Read the model definition and answer for the solid it produces. Units are mm, in the model's axes. A direction names the side the tool comes from. Give positions to 0.01 mm unless a question says otherwise; leave off trailing zeros. Order: outer loops, then holes, each group sorted by start corner. A loop starts at its lowest first (then second) coordinate and runs counter-clockwise, first axis right, second up.
```python
from build123d import *

# Parameters (mm, degrees)
F0_R      = 5.6261
F1_DEPTH  = 12.7
F2_R      = 5.6007
F3_DEPTH  = 9.525
F4_R      = 12.7
F4_R_2    = 5.6007
F6_DEPTH  = 6.35
F7_DEPTH  = 6.35
F8_R      = 7.62
F9_DEPTH  = 6.35
F10_DEPTH = 6.35
F11_R     = 1.27


with BuildPart() as f1:
    # F0 (on Top) → F1 (new body)
    with BuildSketch(Plane.XY):
        Circle(F0_R)
    extrude(amount=F1_DEPTH)

    # F2 (on face) → F3 (join)
    with BuildSketch(Plane.XY.offset(12.7)):
        Circle(F2_R)
    extrude(amount=F3_DEPTH)

    # F4 (on face) → F6 (join)
    with BuildSketch(Plane.XY.offset(22.225)):
        Circle(F4_R)
        Circle(F4_R_2, mode=Mode.SUBTRACT)
    extrude(amount=F6_DEPTH)

    # F7 (add): a face of the model
    f7_faces = [f1.faces().sort_by_distance(p)[0] for p in [
        (0, 0, 22.225),
    ]]
    extrude(f7_faces, amount=F7_DEPTH)

    # F8 (on face) → F9 (join)
    with BuildSketch(Plane(origin=(0, 0, 22.225), x_dir=(1, 0, 0), z_dir=(0, 0, -1))):
        Circle(F8_R)
    extrude(amount=F9_DEPTH)

    # F5 (on face) → F10 (join)
    with BuildSketch(Plane.XY.offset(22.225)):
        with BuildLine():
            ThreePointArc((-6.35, -10.9985226281), (-10.9985226281, -6.35), (-12.7, 0))
            Line((-12.7, 0), (-29.197504538, -9.524838686))
            ThreePointArc((-29.197504538, -9.524838686), (-27.4960271661, -15.874838686), (-22.847504538, -20.523361314))
            Line((-22.847504538, -20.523361314), (-6.35, -10.9985226281))
        make_face()
        with BuildLine():
            Line((-6.35, 30.0482), (-6.35, 10.9985226281))
            ThreePointArc((-6.35, 10.9985226281), (0, 12.7), (6.35, 10.9985226281))
            Line((6.35, 10.9985226281), (6.35, 30.0482))
            ThreePointArc((6.35, 30.0482), (0, 31.7496773719), (-6.35, 30.0482))
        make_face()
        with BuildLine():
            Line((29.197504538, -9.524838686), (12.7, 0))
            ThreePointArc((12.7, 0), (10.9985226281, -6.35), (6.35, -10.9985226281))
            Line((6.35, -10.9985226281), (22.847504538, -20.523361314))
            ThreePointArc((22.847504538, -20.523361314), (27.4960271661, -15.874838686), (29.197504538, -9.524838686))
        make_face()
    extrude(amount=F10_DEPTH)

    # F11
    f11_edges = [f1.edges().sort_by_distance(p)[0] for p in [
        (6.35, 20.523361, 28.575),
        (20.948752, -4.762419, 28.575),
        (27.496027, -15.874839, 28.575),
        (14.598752, -15.760942, 28.575),
        (0, 31.749677, 28.575),
        (-6.35, 20.523361, 28.575),
        (-20.948752, -4.762419, 28.575),
        (-14.598752, -15.760942, 28.575),
        (-27.496027, -15.874839, 28.575),
        (-27.496027, -15.874839, 22.225),
        (-20.948752, -4.762419, 22.225),
        (-6.35, 20.523361, 22.225),
        (0, 31.749677, 22.225),
        (6.35, 20.523361, 22.225),
        (20.948752, -4.762419, 22.225),
        (27.496027, -15.874839, 22.225),
        (14.598752, -15.760942, 22.225),
        (-14.598752, -15.760942, 22.225),
        (-10.998523, 6.35, 22.225),
        (0, -12.7, 22.225),
        (10.998523, 6.35, 22.225),
        (10.998523, 6.35, 28.575),
        (-10.998523, 6.35, 28.575),
        (0, -12.7, 28.575),
    ]]
    fillet(f11_edges, radius=F11_R)


solid = f1.part
```
1) Given pin 1 (1 mm diameter, centred on x = 19, z = 21.5, fed in from +Y); pin 2 (17 mm diameter, centred on x = -2, y = -2, fed in from -Z); pin 3 (5 mm diameter, centred on x = -10, z = 24.5, fed in from -Y); pin 4 (2 mm diameter, centred on y = -3, z = 8.5, fed in from -X), each flat-ended and moving along its own axis, determine where each tip first touches the part or whether it passes through.
Final values:
pin 1: passes through
pin 2: stops at z = 0
pin 3: stops at y = -14.55
pin 4: stops at x = -5.26
2) A tool of negligible diameter and unlimited length cuts with its end or side. For faces 5 (the face through (-1.65, 7.44, 19.09)), 6 (the face through (-14.341, -15.171, 28.213)), 7 (the face through (5.97, 20.28, 28.21)), from which of +Z, -Z, +X, -X, +Y, -Y can it reach the whole face along a straight path? Write none if from no direction.
Final values:
face 5: -Z
face 6: +Z, -Y
face 7: +Z, +X, +Y
3) The part is cut by section A-A on z = 25. Determine the outline of the cut face in (x, y), and give its area (3 significant figures).
Final values:
outline: (-29.2, -9.52) arc R12.7 ccw to (-22.85, -20.52) - (-6.35, -11) arc R12.7 ccw to (6.35, -11) - (22.85, -20.52) arc R12.7 ccw to (29.2, -9.52) - (12.7, 0) arc R12.7 ccw to (6.35, 11) - (6.35, 30.05) arc R12.7 ccw to (-6.35, 30.05) - (-6.35, 11) arc R12.7 ccw to (-12.7, 0) - close
area: 1,230 mm2
4) For a pull along X with two mould halves and no side action, classify faces 1 (the face through (-27.542, -15.794, 25.373)), 2 (the face through (14.58, -15.31, 22.59)), 3 (the face through (20.319, -4.817, 22.607)), 4 (the face through (14.58, -15.31, 28.21)) as released by +X, released by -X, zero draft, split by the parting line, or undercut.
Final values:
face 1: released by -X
face 2: undercut
face 3: released by +X
face 4: undercut
5) The part is cut by section C-C on x = 0. Determine the outline of the cut face in (y, z) (3 decimals).
Final values:
outline: (-12.7, 23.495) arc R1.27 ccw to (-11.43, 22.225) - (-7.62, 22.225) - (-7.62, 15.875) - (-5.601, 15.875) - (-5.601, 12.7) - (-5.626, 12.7) - (-5.626, 0) - (5.626, 0) - (5.626, 12.7) - (5.601, 12.7) - (5.601, 15.875) - (7.62, 15.875) - (7.62, 22.225) - (30.48, 22.225) arc R1.27 ccw to (31.75, 23.495) - (31.75, 27.305) arc R1.27 ccw to (30.48, 28.575) - (-11.43, 28.575) arc R1.27 ccw to (-12.7, 27.305) - close
6) The part is cut by section D-D on z = 5.5. Determine the outline of the cut face in (x, y), and give its area (3 significant figures).
Final values:
outline: circle Ø11.25 at (0, 0)
area: 99.4 mm2
7) Consider L1, parallel to Z at x = -6.5, y = -1 (3 decimals); L2, parallel to Z at x = -7, y = -5.5 (3 decimals); L3, parallel to X at y = -5, z = 15.5. Determine where each line is inside the solid, lowest interval first.
Final values:
L1: z = 15.875 to 28.575
L2: z = 22.225 to 28.575
L3: x = -2.52 to 2.52
8) The part is cut by section B-B on y = 27. Determine the outline of the cut face in (x, z) (3 decimals), and give its area (3 significant figures).
Final values:
outline: (-6.35, 23.495) arc R1.27 ccw to (-5.08, 22.225) - (5.08, 22.225) arc R1.27 ccw to (6.35, 23.495) - (6.35, 27.305) arc R1.27 ccw to (5.08, 28.575) - (-5.08, 28.575) arc R1.27 ccw to (-6.35, 27.305) - close
area: 79.3 mm2
